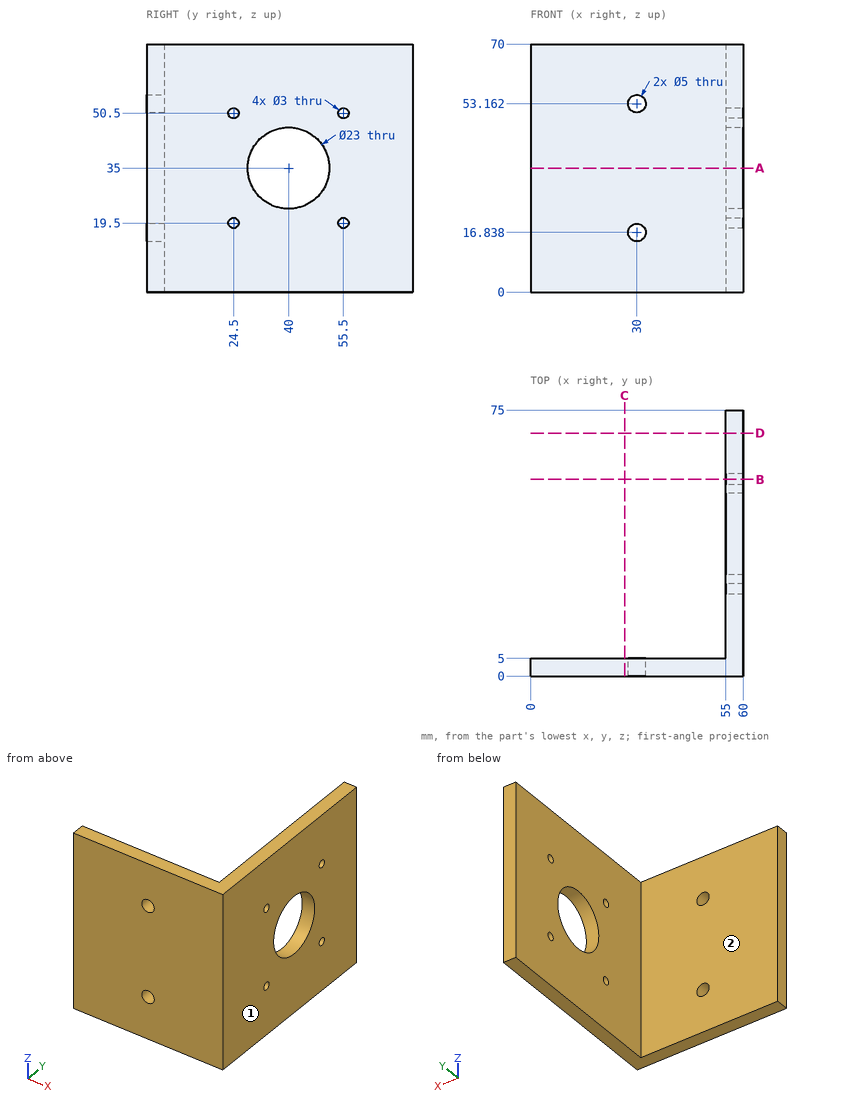
Design review of the part shown in the three views and the two pictorial views. Dimensions are in mm from the part's minimum x, y and z. A direction names the side the tool comes from. Round coordinates to 2 decimals unless told otherwise and drop trailing zeros. Order: outer loops, then holes, each group sorted by start corner. A loop starts at its lowest first (then second) coordinate and runs counter-clockwise, first axis right, second up.
Q1. We need section D-D, the plane y = 68.5. Give the boundary of the cut face in (x, z).
Findings below:
outline: (55, 0) - (60, 0) - (60, 70) - (55, 70) - close
Q2. We need section C-C, the plane x = 26.5. Give the boundary of the cut face in (y, z), plus the area to 3 significant figures.
Findings below:
outline: (0, 0) - (5, 0) - (5, 70) - (0, 70) - close
area: 350 mm2
Q3. Insertion check: P1, Ø4, axis at x = 26, z = 26, coming from the +Y side; P2, Ø20.5, axis at y = 40, z = 35, coming from the -X side; P3, Ø2, axis at y = 38.5, z = 9, coming from the -X side. Each pin has a flat end and moves straight along its axis. Give the tip position at first contact, or say it passes through.
Findings below:
P1: stops at y = 5
P2: passes through
P3: stops at x = 55
Q4. Machinability: for the marked faces 1 and 2, which of the approach directions +Z, -Z, +X, -X, +Y, -Y give a long, thin tool a straight path to every point of the face, cutting with its end or side? Answer none if there is none.
Findings below:
face 1: +Z, -Z, +X, +Y, -Y
face 2: +Z, -Z, -X, +Y
Q5. We need section A-A, the plane z = 35. Give the boundary of the cut face in (x, y), plus the area to 3 significant figures.
Findings below:
outline: (0, 0) - (60, 0) - (60, 28.5) - (55, 28.5) - (55, 5) - (0, 5) - close; (55, 51.5) - (60, 51.5) - (60, 75) - (55, 75) - close
area: 535 mm2
Q6. We need section B-B, the plane y = 55.5. Give the boundary of the cut face in (x, z), plus the area to 3 significant figures.
Findings below:
outline: (55, 0) - (60, 0) - (60, 18) - (55, 18) - close; (55, 21) - (60, 21) - (60, 49) - (55, 49) - close; (55, 52) - (60, 52) - (60, 70) - (55, 70) - close
area: 320 mm2
Q7. Wall thickness on line 1 (Y direction, x = 58.25, z = 50.5); line 2 (X direction, y = 52, z = 25); line 3 (Y direction, x = 27, z = 18): over which ranges is each line inside the solid? List them lowest first.
Findings below:
line 1: y = 0 to 23, 26 to 54, 57 to 75
line 2: x = 55 to 60
line 3: y = 0 to 5
